from build123d import *

# Parameters (mm, degrees)
BOSS_EXTRUDE1_DEPTH     = 5.4
M12X1_75_TAPPED_HOLE1_D = 10.2


with BuildPart() as part:
    # Sketch1 → Boss-Extrude1 (new, symmetric)
    with BuildSketch(Plane(origin=(0, 0, 0), x_dir=(1, 0, 0), z_dir=(0, 1, 0))):
        Polygon((10.392304845, 0), (5.196152423, 9), (-5.196152423, 9), (-10.392304845, 0), (-5.196152423, -9), (5.196152423, -9), align=None)
    extrude(amount=BOSS_EXTRUDE1_DEPTH, both=True)

    # Sketch2 → Cut-Revolve1 (revolve, cut)
    with BuildSketch(Plane(origin=(0, 0, 0), x_dir=(0, 0, -1), z_dir=(1, 0, 0))):
        Polygon((9, 5.4), (13.81357482, 5.4), (13.81357482, 2.620881282), align=None)
    cut_revolve1 = revolve(axis=Axis((0, 0, 0), (0, -1, 0)), mode=Mode.SUBTRACT)

    # Mirror1: Cut-Revolve1 across plane
    add(cut_revolve1.mirror(Plane.ZX), mode=Mode.SUBTRACT)

    # M12x1.75 Tapped Hole1 (through all)
    with Locations(Plane(origin=(0, 5.4, 0), x_dir=(1, 0, 0), z_dir=(0, 1, 0))):
        with Locations((0, 0)):
            Hole(M12X1_75_TAPPED_HOLE1_D / 2)


solid = part.part
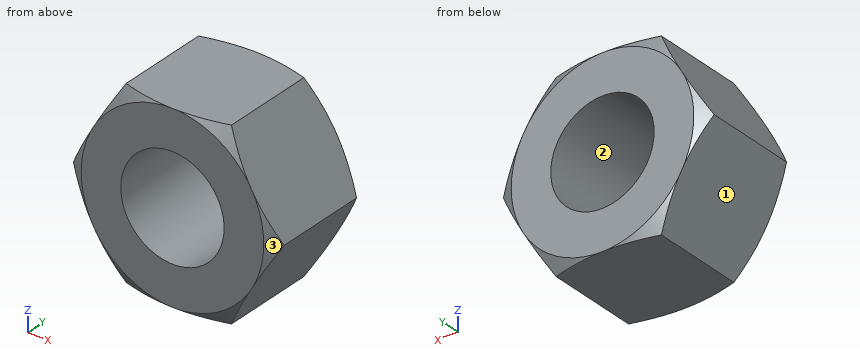
For this review, take the finished solid that the model builds, in its own axes (mm). Face numbers are marked on the shaded views. Give positions to 0.01 mm unless a question says otherwise; leave off trailing zeros. Loops run counter-clockwise (first coordinate to the right, second up) from the corner with the lowest first, then second, coordinate; pieces in that order, holes last. Notation, with made-up numbers: M 73.25,36.25 L 95.25,36.25 A24 cw 95.25,73.25 Z; hole C -39,27.25 d9. An arc over 180 degrees is marked long. Answer as a JSON object with one key per item and string values. Group by question number.
Q1. Add section A-A on y = -1. Give the boundary of the cut face in (x, z), and give its area (3 significant figures).
Q2. Mouldability with a two-part tool opening along Z and no side actions: class the marked faces 1, 2 and 3 as +Z half, -Z half, draft (parallel to the pull), parting line (faces both ways), or undercut.
Q3. Insertion check: P1, Ø1, axis at x = -7.5, y = 1, coming from the -Z side; P2, Ø2, axis at y = 3.5, z = 3.5, coming from the -X side. Each pin has a flat end and moves straight along its axis. Give the tip position at first contact, or say it passes through.
Q4. For probe 1 along X at (y, z) = (-0.5, 1.5); probe 2 along X at (y, z) = (2.75, 3.5); probe 3 along Z at (x, y) = (2.5, 0.5), list the stretches that pass through material, from the lowest coordinate up. Write a range as [from, to].
Checked values:
{
 "1": {"outline": "M -10.39,0 L -5.2,-9 L 5.2,-9 L 10.39,0 L 5.2,9 L -5.2,9 Z; hole C 0,0 d10.2", "area": "199 mm²"},
 "2": {"face 1": "-Z half", "face 2": "undercut", "face 3": "parting line"},
 "3": {"P1": "z = -5.88", "P2": "x = -8.95"},
 "4": {"probe 1": "[-9.53, -4.87], [4.87, 9.53]", "probe 2": "[-8.37, -3.71], [3.71, 8.37]", "probe 3": "[-9, -4.45], [4.45, 9]"}
}
